Input: dimensioned drawing with shaded views. Units: mm. Origin: part minimum x, y, z. A direction names the side the tool comes from. Coordinates: 2 decimals unless noted, no trailing zeros. Order: outer loops, then holes, each group sorted by start corner. A loop starts at its lowest first (then second) coordinate and runs counter-clockwise, first axis right, second up. Notation, with made-up numbers: (58, -16) -> (109, -16) arc R21 cw to (109, -8) -> close; hole circle Ø8 at (-30.75, 5). An arc over 180 degrees is marked (long way). Write item = value, one per line. Start each with the question number.
Item 1: Section query B-B (z = 7). Output: boundary loops of the cut face in (x, y).
Item 2: Section query A-A (y = 7.5). Output: boundary loops of the cut face in (x, z).
Item 3: Contact query for flat-ended pins moving along their axis: pin 1 (5 mm diameter, centred on x = 8.5, z = 3, fed in from -Y); pin 2 (6 mm diameter, centred on x = 1.5, y = 3.5, fed in from -Z); pin 3 (1 mm diameter, centred on x = 7, y = 5.5, fed in from -Z); pin 4 (4 mm diameter, centred on y = 1.5, z = 4.5, fed in from +X). Output: stop coordinate, or through.
Item 4: Ray query, line 1 along Z through (x, y) = (7, 8.75); line 2 along Z through (x, y) = (7, 0.9); line 3 along Y through (x, z) = (8.75, 12). Return the intervals inside material, ascending. Write a range as [from, to].
Item 5: Set-up query: the marked faces 1, 2 and 3. Return all of +Z, -Z, +X, -X, +Y, -Y with unobstructed straight access to the full face (end or side cutting, diameter ignored); none if empty.
Item 6: Mould query, pull axis X, two halves, no side actions, for the marked faces 4, 5 and 6. Classes: released by +X, released by -X, zero draft, split by the parting line, or undercut.
Item 7: Section query D-D (y = 3.5). Output: boundary loops of the cut face in (x, z), then the cut area to 3 significant figures.
Item 8: Section query C-C (x = 7). Output: boundary loops of the cut face in (y, z), then the cut area to 3 significant figures.
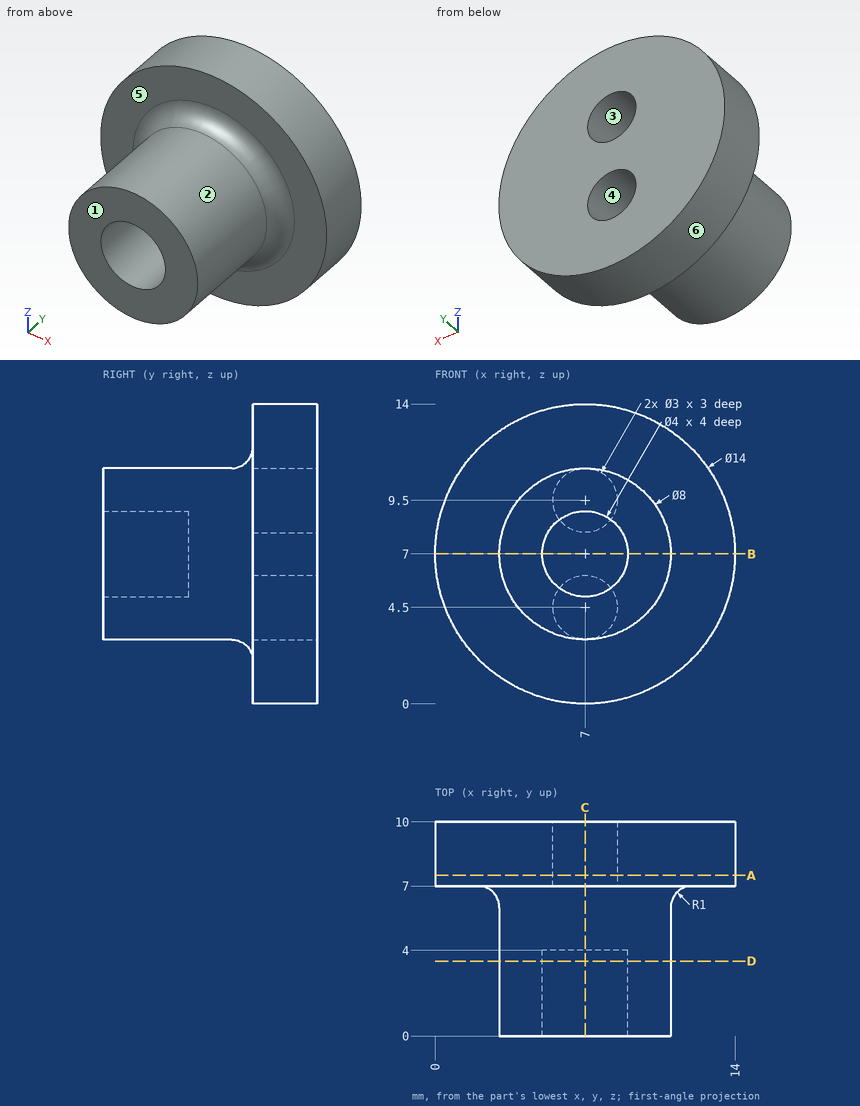
Computed:
q1.outline = (0, 7) -> (2, 7) arc R1 cw to (3, 6) -> (3, 0) -> (5, 0) -> (5, 4) -> (9, 4) -> (9, 0) -> (11, 0) -> (11, 6) arc R1 cw to (12, 7) -> (14, 7) -> (14, 10) -> (0, 10) -> close
q2.outline = circle Ø14 at (7, 7); hole circle Ø3 at (7, 4.5); hole circle Ø3 at (7, 9.5)
q3.pin_1 = 0
q3.pin_2 = 3.88
q3.pin_3 = 3
q3.pin_4 = 10.97
q4.line_1 = [0, 3], [6, 8], [11, 14]
q4.line_2 = [3, 5], [9, 11]
q4.line_3 = [7, 10]
q5.face_1 = +Z, -Z, +X, -X, -Y
q5.face_2 = -Y
q5.face_3 = +Y
q6.face_4 = undercut
q6.face_5 = zero draft
q6.face_6 = split by the parting line
q7.outline = circle Ø8 at (7, 7); hole circle Ø4 at (7, 7)
q7.area = 37.7 mm^2
q8.outline = (0, 3) -> (6, 3) arc R1 cw to (7, 2) -> (7, 0) -> (10, 0) -> (10, 3) -> (7, 3) -> (7, 6) -> (10, 6) -> (10, 8) -> (7, 8) -> (7, 11) -> (10, 11) -> (10, 14) -> (7, 14) -> (7, 12) arc R1 cw to (6, 11) -> (0, 11) -> (0, 9) -> (4, 9) -> (4, 5) -> (0, 5) -> close
q8.area = 64.4 mm^2
